```python
from build123d import *

# Parameters (mm, degrees)
SKETCH1_R           = 1.25
SKETCH1_R_2         = 3
BOSS_EXTRUDE2_DEPTH = 2
FILLET1_R           = 1
CUT_EXTRUDE1_DEPTH  = 2
BOSS_EXTRUDE3_DEPTH = 2


with BuildPart() as part:
    # Sketch1 → Boss-Extrude2 (new body)
    with BuildSketch(Plane(origin=(0, 0, 0), x_dir=(1, 0, 0), z_dir=(0, 1, 0))):
        with BuildLine():
            Line((507.5, -879.015784841), (572.5, -991.599087333))
            ThreePointArc((572.5, -991.599087333), (308.404936897, -1102.683723875), (25, -1144.7270417))
            Line((25, -1144.7270417), (25, -1165))
            Line((25, -1165), (-25, -1165))
            Line((-25, -1165), (-25, -1144.7270417))
            ThreePointArc((-25, -1144.7270417), (-308.404936897, -1102.683723875), (-572.5, -991.599087333))
            Line((-572.5, -991.599087333), (-507.5, -879.015784841))
            ThreePointArc((-507.5, -879.015784841), (-274.756394269, -977.104868378), (-25, -1014.692071517))
            Line((-25, -1014.692071517), (-25, -995))
            Line((-25, -995), (25, -995))
            Line((25, -995), (25, -1014.692071517))
            ThreePointArc((25, -1014.692071517), (274.756394269, -977.104868378), (507.5, -879.015784841))
        make_face()
        with Locations((-17, -1005)):
            Circle(SKETCH1_R, mode=Mode.SUBTRACT)
        with Locations((17, -1005)):
            Circle(SKETCH1_R, mode=Mode.SUBTRACT)
        with Locations((502.839745962, -890.943988071)):
            Circle(SKETCH1_R_2, mode=Mode.SUBTRACT)
        with Locations((559.839745962, -989.670884103)):
            Circle(SKETCH1_R_2, mode=Mode.SUBTRACT)
        with Locations((480.404221067, -1030.524519059)):
            Circle(SKETCH1_R_2, mode=Mode.SUBTRACT)
        with Locations((432.237043229, -927.200160947)):
            Circle(SKETCH1_R_2, mode=Mode.SUBTRACT)
        with Locations((-17, -1155)):
            Circle(SKETCH1_R, mode=Mode.SUBTRACT)
        with Locations((17, -1155)):
            Circle(SKETCH1_R, mode=Mode.SUBTRACT)
        with Locations((177.531862859, -1007.477760385)):
            Circle(SKETCH1_R_2, mode=Mode.SUBTRACT)
        with Locations((197.315472209, -1119.748009343)):
            Circle(SKETCH1_R_2, mode=Mode.SUBTRACT)
        with Locations((-559.839745962, -989.670884103)):
            Circle(SKETCH1_R_2, mode=Mode.SUBTRACT)
        with Locations((-502.839745962, -890.943988071)):
            Circle(SKETCH1_R_2, mode=Mode.SUBTRACT)
        with Locations((-480.404221067, -1030.524519059)):
            Circle(SKETCH1_R_2, mode=Mode.SUBTRACT)
        with Locations((-432.237043229, -927.200160947)):
            Circle(SKETCH1_R_2, mode=Mode.SUBTRACT)
        with Locations((-197.315472209, -1119.748009343)):
            Circle(SKETCH1_R_2, mode=Mode.SUBTRACT)
        with Locations((-177.531862859, -1007.477760385)):
            Circle(SKETCH1_R_2, mode=Mode.SUBTRACT)
    extrude(amount=BOSS_EXTRUDE2_DEPTH)

    # Fillet1
    fillet1_edges = [part.edges().sort_by_distance(p)[0] for p in [
        (25, 1, 1165),
        (-25, 1, 1165),
        (-572.5, 1, 991.599087333),
        (-507.5, 1, 879.015784841),
        (-25, 1, 995),
        (25, 1, 995),
        (507.5, 1, 879.015784841),
        (572.5, 1, 991.599087333),
    ]]
    fillet(fillet1_edges, radius=FILLET1_R)

    # Sketch3 → Cut-Extrude1 (cut)
    with BuildSketch(Plane(origin=(0, 2, 0), x_dir=(1, 0, 0), z_dir=(0, 1, 0))):
        with BuildLine():
            Line((519.871701126, -931.945073732), (527.997692321, -914.518829378))
            Line((527.997692321, -914.518829378), (552.001843085, -956.095238095))
            Line((552.001843085, -956.095238095), (532.847277184, -954.419430724))
            ThreePointArc((532.847277184, -954.419430724), (529.319600421, -955.471006493), (527.467771352, -958.652365329))
            ThreePointArc((527.467771352, -958.652365329), (485.99383482, -966.487373624), (513.516119308, -934.48739514))
            ThreePointArc((513.516119308, -934.48739514), (517.197171414, -934.474343541), (519.871701126, -931.945073732))
        make_face()
    extrude(amount=-CUT_EXTRUDE1_DEPTH, mode=Mode.SUBTRACT)

    # Sketch4 → Boss-Extrude3 (add)
    with BuildSketch(Plane(origin=(0, 2, 0), x_dir=(1, 0, 0), z_dir=(0, 1, 0))):
        with BuildLine():
            Line((-547.152258221, -916.194636749), (-527.997692321, -914.518829378))
            Line((-527.997692321, -914.518829378), (-552.001843085, -956.095238095))
            Line((-552.001843085, -956.095238095), (-560.12783428, -938.668993741))
            ThreePointArc((-560.12783428, -938.668993741), (-562.802363992, -936.139723932), (-566.483416097, -936.126672333))
            ThreePointArc((-566.483416097, -936.126672333), (-594.005700585, -904.126693849), (-552.531764054, -911.961702144))
            ThreePointArc((-552.531764054, -911.961702144), (-550.679934984, -915.14306098), (-547.152258221, -916.194636749))
        make_face()
        with BuildLine():
            Line((5.48633271, -986.815018385), (7.679491924, -995))
            Line((7.679491924, -995), (-7.679491924, -995))
            Line((-7.679491924, -995), (-5.48633271, -986.815018385))
            ThreePointArc((-5.48633271, -986.815018385), (-5.549842721, -985.31863757), (-6.457260037, -984.127091147))
            ThreePointArc((-6.457260037, -984.127091147), (0, -963.819660113), (6.457260037, -984.127091147))
            ThreePointArc((6.457260037, -984.127091147), (5.549842721, -985.31863757), (5.48633271, -986.815018385))
        make_face()
        with BuildLine():
            Line((-7.679491924, -1165), (7.679491924, -1165))
            Line((7.679491924, -1165), (5.48633271, -1173.184981615))
            ThreePointArc((5.48633271, -1173.184981615), (5.549842721, -1174.68136243), (6.457260037, -1175.872908853))
            ThreePointArc((6.457260037, -1175.872908853), (0, -1196.180339887), (-6.457260037, -1175.872908853))
            ThreePointArc((-6.457260037, -1175.872908853), (-5.549842721, -1174.68136243), (-5.48633271, -1173.184981615))
            Line((-5.48633271, -1173.184981615), (-7.679491924, -1165))
        make_face()
    extrude(amount=-BOSS_EXTRUDE3_DEPTH)


solid = part.part
```
Geometry: final body of the model. Coordinates: model frame, mm. A direction names the side the tool comes from. Round coordinates to 2 decimals unless told otherwise and drop trailing zeros. Order: outer loops, then holes, each group sorted by start corner. A loop starts at its lowest first (then second) coordinate and runs counter-clockwise, first axis right, second up. Notation, with made-up numbers: (-27, 61.5) -> (-6, 61.5) arc R31 cw to (-6, 86.5) -> close; hole circle Ø4 at (29, 77.25). An arc over 180 degrees is marked (long way). Use one line per item in the form item = value. Start each with the question number.
1. Draft query along Z for faces 1 (the face through (-4, 0, 1036)), 2 (the face through (-0.395, 1.014, 963.827)), 3 (the face through (-277.68, 0.99, 976.28)), 4 (the face through (486.39, 1.01, 967.15)). Return one class per face: pulls with the +Z half, pulls with the -Z half, needs draft (parallel to the pull), parting line crosses it, or undercut.
2. Cut plane B-B (x = -255). Return the cut outline in (y, z), then the cut area to 3 significant figures.
3. Cut plane C-C (y = 1.4). Count the separate pieces of the cut face and the enclosed holes in it, then the cut area to 3 significant figures.
4. Reachability of faces 5 (the face through (-518.139, 0.986, 897.443)), 6 (the face through (-594.38, 1.01, 904.8)), 7 (the face through (-562.141, 0.986, 973.656)) from +Z, -Z, +X, -X, +Y, -Y: full face, straight path, thin tool, end or side. Return the list, or none.
5. Cut plane A-A (z = 1079). Return the cut outline in (x, y).
6. Line query: probe 1 along Z at (x, y) = (-17, 1.1); probe 2 along X at (y, z) = (0.6, 1155); probe 3 along X at (y, z) = (0.6, 1153). Output: solid intervals per line, ascending.
Solution:
q1.face_1 = needs draft
q1.face_2 = undercut
q1.face_3 = pulls with the -Z half
q1.face_4 = undercut
q2.outline = (0, 982.45) -> (2, 982.45) -> (2, 1116.24) -> (0, 1116.24) -> close
q2.area = 268 mm^2
q3.separate_pieces = 1
q3.enclosed_holes = 16
q3.area = 150,000 mm^2
q4.face_5 = -Z, +Y, -Y
q4.face_6 = +Y, -Y
q4.face_7 = -X, +Y, -Y
q5.outline = (-383.12, 0) -> (383.12, 0) -> (383.12, 2) -> (-383.12, 2) -> close
q6.probe_1 = 995 to 1003.75, 1006.25 to 1153.75, 1156.25 to 1165
q6.probe_2 = -25 to -18.25, -15.75 to 15.75, 18.25 to 25
q6.probe_3 = -25 to 25
